Could you check a few things on this model? Use its own coordinates, in mm. A direction names the side the tool comes from. Coordinates: 2 decimals unless noted, no trailing zeros. Loops run counter-clockwise (first coordinate to the right, second up) from the corner with the lowest first, then second, coordinate; pieces in that order, holes last. Notation, with made-up numbers: M -28.5,-19 L 15.5,-19 A27 ccw 15.5,-1 Z; hole C -17.75,-14 d2. An arc over 180 degrees is marked long. Write each question's results on one line, items separated by ' | '.
```python
from build123d import *

# Parameters (mm, degrees)
F1_DEPTH = 3


with BuildPart() as f1:
    # F0 (on Front) → F1 (new body)
    with BuildSketch(Plane.XZ):
        with BuildLine():
            Line((10, -19.17), (10, 19.17))
            Line((10, 19.17), (1.5, 19.17))
            Line((1.5, 19.17), (1.5, -4.28))
            Line((1.5, -4.28), (-1.5, -4.28))
            Line((-1.5, -4.28), (-1.5, 19.17))
            Line((-1.5, 19.17), (-10, 19.17))
            Line((-10, 19.17), (-10, -19.17))
            ThreePointArc((-10, -19.17), (0, -29.17), (10, -19.17))
        make_face()
    extrude(amount=F1_DEPTH)


solid = f1.part
```
(1) Imagine slicing it at B-B, the plane y = -1.25. List the corners of the cut face in (x, z) for me, and give its area (3 significant figures).
Reported:
outline: M -10,-19.17 A10 ccw 10,-19.17 L 10,19.17 L 1.5,19.17 L 1.5,-4.28 L -1.5,-4.28 L -1.5,19.17 L -10,19.17 Z | area: 854 mm2
(2) Which directions (+Z, -Z, +X, -X, +Y, -Y) give clear straight access to the entire face, cutting with the end or side of a thin tool? Please do faces 4 (the flat face through (-10, -1, 0)), 5 (the flat face through (0, -1, -4.28)).
Reported:
face 4: +Z, -Z, -X, +Y, -Y | face 5: +Z, +Y, -Y
(3) If we mould it in two halves opening along X, with no side actions, what happens to faces 1 (the flat face through (10, -1, 0)), 2 (the flat face through (6, -1, 19.17)), 3 (the flat face through (-1.5, -1, 7))? For each: released by +X, released by -X, zero draft, split by the parting line, or undercut.
Reported:
face 1: released by +X | face 2: zero draft | face 3: undercut
(4) Imagine slicing it at D-D, the plane x = 4. List the corners of the cut face in (y, z) for me.
Reported:
outline: M -3,-28.34 L 0,-28.34 L 0,19.17 L -3,19.17 Z
(5) Imagine slicing it at C-C, the plane x = 0. List the corners of the cut face in (y, z) for me, and give its area (3 significant figures).
Reported:
outline: M -3,-29.17 L 0,-29.17 L 0,-4.28 L -3,-4.28 Z | area: 74.7 mm2
(6) Imagine slicing it at A-A, the plane z = -0.5. List the corners of the cut face in (x, y) for me, and give its area (3 significant figures).
Reported:
outline: M -10,-3 L -1.5,-3 L -1.5,0 L -10,0 Z; M 1.5,-3 L 10,-3 L 10,0 L 1.5,0 Z | area: 51.0 mm2
(7) Please list where these lines run through material, in increasing order: probe 1 along X at (y, z) = (-1.1, 7); probe 2 along Z at (x, y) = (0.25, -0.6); probe 3 along Z at (x, y) = (-5.25, -1.45). Write a range as from..to.
Reported:
probe 1: x = -10..-1.5, 1.5..10 | probe 2: z = -29.17..-4.28 | probe 3: z = -27.68..19.17
